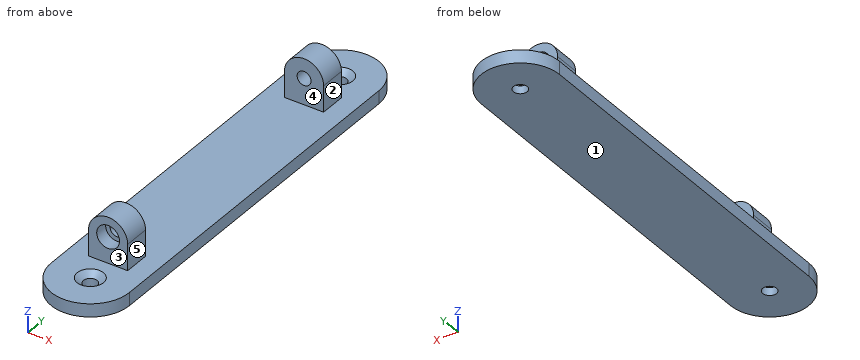
from build123d import *

# Parameters (mm, degrees)
BOSS_EXTRUDE1_DEPTH                                 = 6.35
CSK_FOR_1_4_FLAT_HEAD_MACHINE_SCREW_100_D           = 6.7564
CSK_FOR_1_4_FLAT_HEAD_MACHINE_SCREW_100_CSINK_D     = 12.8778
CSK_FOR_1_4_FLAT_HEAD_MACHINE_SCREW_100_CSINK_ANGLE = 100
SKETCH5_W                                           = 19.05
SKETCH5_H                                           = 12.7
BOSS_EXTRUDE2_DEPTH                                 = 12.7
BOSS_EXTRUDE3_DEPTH                                 = 12.7
CBORE_FOR_1_4_SOCKET_HEAD_CAP_SCREW1_D              = 6.7564
CBORE_FOR_1_4_SOCKET_HEAD_CAP_SCREW1_DEPTH          = 12.7
CBORE_FOR_1_4_SOCKET_HEAD_CAP_SCREW1_CBORE_D        = 11.1125
CBORE_FOR_1_4_SOCKET_HEAD_CAP_SCREW1_CBORE_DEPTH    = 6.35
CBORE_FOR_1_4_SOCKET_HEAD_CAP_SCREW1_TIP            = 2.029827343


with BuildPart() as part:
    # Sketch1 → Boss-Extrude1 (new body)
    with BuildSketch(Plane.XY):
        with BuildLine():
            Line((0, 0), (38.1, 0))
            Line((38.1, 0), (38.1, 88.9))
            ThreePointArc((38.1, 88.9), (19.05, 107.95), (0, 88.9))
            Line((0, 88.9), (0, 0))
        make_face()
    extrude(amount=BOSS_EXTRUDE1_DEPTH)

    # CSK for 1/4 Flat Head Machine Screw (100)1 (through all)
    with Locations(Plane.XY.offset(6.35)):
        with Locations((19.05, 88.9)):
            CounterSinkHole(CSK_FOR_1_4_FLAT_HEAD_MACHINE_SCREW_100_D / 2, CSK_FOR_1_4_FLAT_HEAD_MACHINE_SCREW_100_CSINK_D / 2, counter_sink_angle=CSK_FOR_1_4_FLAT_HEAD_MACHINE_SCREW_100_CSINK_ANGLE)

    # Sketch5 → Boss-Extrude2 (add)
    with BuildSketch(Plane.XY.offset(6.35)):
        with Locations((19.05, 69.85)):
            Rectangle(SKETCH5_W, SKETCH5_H)
    extrude(amount=BOSS_EXTRUDE2_DEPTH)

    # Sketch6 → Boss-Extrude3 (add)
    with BuildSketch(Plane(origin=(0, 76.2, 0), x_dir=(1, 0, 0), z_dir=(0, 1, 0))):
        with BuildLine():
            Line((9.525, -19.05), (28.575, -19.05))
            ThreePointArc((28.575, -19.05), (19.05, -28.575), (9.525, -19.05))
        make_face()
    extrude(amount=-BOSS_EXTRUDE3_DEPTH)

    # CBORE for 1/4 Socket Head Cap Screw1
    with Locations(Plane(origin=(0, 76.2, 0), x_dir=(1, 0, 0), z_dir=(0, 1, 0))):
        with Locations((19.05, -19.05)):
            CounterBoreHole(CBORE_FOR_1_4_SOCKET_HEAD_CAP_SCREW1_D / 2, CBORE_FOR_1_4_SOCKET_HEAD_CAP_SCREW1_CBORE_D / 2, CBORE_FOR_1_4_SOCKET_HEAD_CAP_SCREW1_CBORE_DEPTH, depth=CBORE_FOR_1_4_SOCKET_HEAD_CAP_SCREW1_DEPTH)
            with Locations((0, 0, -(CBORE_FOR_1_4_SOCKET_HEAD_CAP_SCREW1_DEPTH + CBORE_FOR_1_4_SOCKET_HEAD_CAP_SCREW1_TIP / 2))):  # 118° drill point
                Cone(0, CBORE_FOR_1_4_SOCKET_HEAD_CAP_SCREW1_D / 2, CBORE_FOR_1_4_SOCKET_HEAD_CAP_SCREW1_TIP, mode=Mode.SUBTRACT)

    # Mirror1: part across plane


with BuildPart() as part_1:
    add(part.part)
    add(part.part.mirror(Plane(origin=(0, 0, 6.35), x_dir=(0, 0, 1), z_dir=(0, 1, 0))))


solid = part_1.part
The model under review builds one solid part; all positions refer to its coordinate system, in mm. Face numbers are marked on the shaded views. A direction names the side the tool comes from. Coordinates: 2 decimals unless noted, no trailing zeros. Write each loop counter-clockwise with the first axis right and the second up, starting at its lowest first coordinate (ties: lowest second). Pieces come first, ordered by that corner, then holes. Notation, with made-up numbers: (44.25, 17) - (70.25, 17) arc R19 cw to (70.25, 36) - close; hole circle Ø7 at (64, 73). An arc over 180 degrees is marked (long way). Answer as CSV lines item,"result".
(1) For line 1 along Z through (x, y) = (19.05, 74.5) (3 decimals); line 2 along Y through (x, z) = (25, 25.5); line 3 along Z through (x, y) = (19, -68), list the stretches that pass through material, from the lowest coordinate up. Write a range as [from, to].
Data:
line 1,"z = [0, 13.494], [24.606, 28.575]"
line 2,"y = [-76.2, -63.5], [63.5, 76.2]"
line 3,"z = [0, 15.67], [22.43, 28.57]"
(2) Clearance check with flat-ended pins moving along their axes: pin 1 Ø9 at (x, z) = (19.05, 19.05) entering from +Y; pin 2 Ø3 at (x, y) = (29, 81.5) entering from +Z; pin 3 Ø15 at (x, z) = (15, 14) entering from +Y. State where each tip first meets the part, or that it passes through.
Data:
pin 1,"stops at y = 69.85"
pin 2,"stops at z = 6.35"
pin 3,"stops at y = 76.2"
(3) Mouldability with a two-part tool opening along Y and no side actions: class the marked faces 3, 4 and 5 as pulls with the +Y half, pulls with the -Y half, needs draft (parallel to the pull), parting line crosses it, or undercut.
Data:
face 3,"pulls with the -Y half"
face 4,"undercut"
face 5,"needs draft"
(4) Tool access review of the marked faces 1 and 2: name each direction out of +Z, -Z, +X, -X, +Y, -Y from which nothing blocks a thin tool from reaching the whole face with its end or side.
Data:
face 1,"-Z, +X, -X, +Y, -Y"
face 2,"+Z, +X, +Y, -Y"
(5) We need section A-A (x = 19.05). Count the separate pieces of the cut face and the enclosed holes in it, plus the area to 3 significant figures.
Data:
separate pieces,"5"
enclosed holes,"0"
area,"1,610 mm2"
(6) We need section C-C (x = 33). Give the boundary of the cut face in (y, z), plus the area to 3 significant figures.
Data:
outline,"(-101.87, 0) - (101.87, 0) - (101.87, 6.35) - (-101.87, 6.35) - close"
area,"1,290 mm2"
(7) We need section B-B (y = -17). Give the boundary of the cut face in (x, z).
Data:
outline,"(0, 0) - (38.1, 0) - (38.1, 6.35) - (0, 6.35) - close"
